from build123d import *

# Parameters (mm, degrees)
ESBO_O1_W                  = 38
ESBO_O1_H                  = 38
RESSALTO_EXTRUS_O1_DEPTH   = 15
CORTE_EXTRUS_O1_DEPTH      = 52.28352562
ESBO_O7_W                  = 0.3
ESBO_O7_H                  = 28
ESBO_O7_W_2                = 28
ESBO_O7_H_2                = 0.3
ESBO_O7_W_3                = 2
ESBO_O7_H_3                = 2
CORTE_EXTRUS_O2_DEPTH      = 52.28352562
FURO_DE_DI_METRO_7_0_7_3_D = 5
FURO_DE_DI_METRO_7_0_7_2_D = 5
FILETE1_R                  = 4
FILETE2_R                  = 0.15


with BuildPart() as part:
    # Esboço1 → Ressalto-extrusão1 (new body)
    with BuildSketch(Plane(origin=(10, 0, 0), x_dir=(0, 0, -1), z_dir=(1, 0, 0))):
        with Locations((-12, 19)):
            Rectangle(ESBO_O1_W, ESBO_O1_H)
    extrude(amount=-RESSALTO_EXTRUS_O1_DEPTH)

    # Esboço2 → Corte-extrusão1 (cut, through all)
    with BuildSketch(Plane.ZY.offset(5)):
        Polygon((31, 38), (-1, 38), (-1, 12), (5, 6), (31, 6), align=None)
    extrude(amount=-CORTE_EXTRUS_O1_DEPTH, mode=Mode.SUBTRACT)

    # Esboço7 → Corte-extrusão2 (cut, through all)
    with BuildSketch(Plane(origin=(10, 0, 0), x_dir=(0, 0, -1), z_dir=(1, 0, 0))):
        with Locations((6.85, 19)):
            Rectangle(ESBO_O7_W, ESBO_O7_H)
        with Locations((-12, 0.15)):
            Rectangle(ESBO_O7_W_2, ESBO_O7_H_2)
        with Locations((-13, 5.85)):
            Rectangle(ESBO_O7_W_3, ESBO_O7_H_2)
        with Locations((1.15, 20)):
            Rectangle(ESBO_O7_W, ESBO_O7_H_3)
        with Locations((-18, 5.85)):
            Rectangle(ESBO_O7_W_3, ESBO_O7_H_2)
        with Locations((1.15, 25)):
            Rectangle(ESBO_O7_W, ESBO_O7_H_3)
    extrude(amount=-CORTE_EXTRUS_O2_DEPTH, mode=Mode.SUBTRACT)

    # Furo de diâmetro Ø7.0 (7)3 (through all)
    with Locations(Plane(origin=(0, 6, 0), x_dir=(1, 0, 0), z_dir=(0, 1, 0))):
        with Locations((2.5, -18)):
            Hole(FURO_DE_DI_METRO_7_0_7_3_D / 2)

    # Furo de diâmetro Ø7.0 (7)2 (through all)
    with Locations(Plane(origin=(0, 0, -7), x_dir=(-1, 0, 0), z_dir=(0, 0, -1))):
        with Locations((-2.5, 25)):
            Hole(FURO_DE_DI_METRO_7_0_7_2_D / 2)

    # Filete1
    filete1_edges = [part.edges().sort_by_distance(p)[0] for p in [
        (2.5, 6, 31),
        (2.5, 6, 5),
        (2.5, 12, -1),
        (2.5, 38, -1),
    ]]
    fillet(filete1_edges, radius=FILETE1_R)

    # Filete2
    filete2_edges = [part.edges().sort_by_distance(p)[0] for p in [
        (2.5, 5, -7),
        (2.5, 5, -6.7),
        (2.5, 33, -7),
        (2.5, 33, -6.7),
        (2.5, 0, 26),
        (2.5, 0.3, 26),
        (2.5, 0.3, -2),
        (2.5, 0, -2),
        (2.5, 19, -1.3),
        (2.5, 19, -1),
        (2.5, 21, -1.3),
        (2.5, 21, -1),
        (2.5, 5.7, 14),
        (2.5, 6, 14),
        (2.5, 5.7, 12),
        (2.5, 6, 12),
        (-2.395643924, 26, -1.3),
        (-2.395643924, 24, -1.3),
        (-2.395643924, 24, -1),
        (-2.395643924, 26, -1),
        (-2.395643924, 5.7, 19),
        (-2.395643924, 5.7, 17),
        (-2.395643924, 6, 17),
        (-2.395643924, 6, 19),
    ]]
    fillet(filete2_edges, radius=FILETE2_R - 0.0001)  # a hair under: the kernel refuses the full size


solid = part.part
Could you check a few things on this model? Use its own coordinates, in mm. A direction names the side the tool comes from. Coordinates: 2 decimals unless noted, no trailing zeros. Order: outer loops, then holes, each group sorted by start corner. A loop starts at its lowest first (then second) coordinate and runs counter-clockwise, first axis right, second up. Notation, with made-up numbers: (-9, 62.25) - (41, 62.25) arc R24 ccw to (41, 88.25) - close; hole circle Ø1 at (42, -23). An arc over 180 degrees is marked (long way). Answer in a Markdown table with one row per item. Add a question column.
(1) I need wall thicknesses on L1, parallel to Z at x = 2.5, y = 1.95; L2, parallel to X at y = 4.6, z = 18; L3, parallel to Z at x = 5, y = 16.5. Which ranges of each line are inside material? Lowest first, please.
(2) If we section it at C-C, the plane x = 1: State how many separate pieces and enclosed holes the cut face has, then the cut area to 3 significant figures.
(3) On a 3-axis mill with a long thin cutter (end or side, diameter ignored), from which of +Z, -Z, +X, -X, +Y, -Y can I reach the whole of each face in a straight line? I mean faces 1 (the face through (-2, 5.7, 18)), 2 (the face through (3, 19, -6.7)), 3 (the face through (2, 6, 9)), 4 (the face through (-2, 25, -1.3)). Say none if no direction works.
(4) If we section it at B-B, the plane y = 25: Please give me the cut outline in (x, z), then the cut area to 3 significant figures.
(5) If we section it at A-A, the plane z = 18: Please give me the cut outline in (x, y), then the cut area to 3 significant figures.
(6) If we section it at D-D, the plane y = 9.5: Please give me the cut outline in (x, z), then the cut area to 3 significant figures.
(7) Will these pins go through, and if not, where does the flat tip stop? pin 1 (1.4 mm diameter, centred on x = -3, z = 18, fed in from +Y); pin 2 (1.5 mm diameter, centred on x = 8.5, y = 11.5, fed in from +Z); pin 3 (1.5 mm diameter, centred on x = -1, z = -2, fed in from +Y); pin 4 (6 mm diameter, centred on y = 16, z = 3.5, fed in from -X).
(8) If we mould it in two halves opening along Y, with no side actions, what happens to faces 5 (the face through (3, 2, -7)), 6 (the face through (3, 5.7, 13)), 7 (the face through (7, 25, -1.3))? For each: released by +Y, released by -Y, zero draft, split by the parting line, or undercut.
Results are:
| question | item | result |
|---|---|---|
| 1 | L1 | z = -7 to 15.5, 20.5 to 31 |
| 1 | L2 | x = -5 to 0, 5 to 10 |
| 1 | L3 | z = -6.7 to -1 |
| 2 | separate pieces | 3 |
| 2 | enclosed holes | 0 |
| 2 | area | 368 mm2 |
| 3 | face 1 | +X, -X, +Y |
| 3 | face 2 | -Z, +X, -X |
| 3 | face 3 | +Z, +X, -X, +Y |
| 3 | face 4 | +Z, +X, -X |
| 4 | outline | (-5, -6.7) - (0, -6.7) - (0, -1.3) - (-5, -1.3) - close; (5, -6.7) - (10, -6.7) - (10, -1.3) - (5, -1.3) - close |
| 4 | area | 54.0 mm2 |
| 5 | outline | (-5, 0.3) - (0, 0.3) - (0, 5.7) - (-5, 5.7) - close; (5, 0.3) - (10, 0.3) - (10, 5.7) - (5, 5.7) - close |
| 5 | area | 54.0 mm2 |
| 6 | outline | (-5, -6.7) - (10, -6.7) - (10, 1.5) - (-5, 1.5) - close |
| 6 | area | 123 mm2 |
| 7 | pin 1 | stops at y = 5.7 |
| 7 | pin 2 | stops at z = 0.25 |
| 7 | pin 3 | stops at y = 37.31 |
| 7 | pin 4 | passes through |
| 8 | face 5 | zero draft |
| 8 | face 6 | released by +Y |
| 8 | face 7 | undercut |
